Geometry: see drawing. Coordinates: mm, zero at the bounding-box minimum. Give positions to 0.01 mm unless a question says otherwise; leave off trailing zeros. Write each loop counter-clockwise with the first axis right and the second up, starting at its lowest first coordinate (ties: lowest second). Pieces come first, ordered by that corner, then holes. Notation, with made-up numbers: M -16,80 L 14,80 A18 cw 14,107 Z; hole C 78.25,-2.75 d2. An arc over 180 degrees is marked long. Use a Markdown table: item, result. Add a question column.
1) Section B-B on z = 1.8. Return the cut outline in (x, y) (1 decimal).
2) Pin query (flat end, axial travel): pin 1 (1 mm diameter, centred on x = 4.5, z = 0.5, fed in from +Y) (1 decimal); pin 2 (3.5 mm diameter, centred on x = 3, y = 3, fed in from +Z); pin 3 (2.5 mm diameter, centred on x = 8, y = 11, fed in from +Z). Return the tip coordinate at first contact, or that it passes through.
3) Section A-A on y = 3. Return the cut outline in (x, z), then the cut area to 3 significant figures.
4) Section C-C on x = 7.25. Return the cut outline in (y, z), then the cut area to 3 significant figures.
5) Draft query along Y for the marked faces 1, 2 and 3. Return one class per face: +Y half, -Y half, draft (parallel to the pull), parting line (faces both ways), or undercut.
6) Section D-D on y = 11. Return the cut outline in (x, z).
7) Line query: line 1 (X direction, y = 4, z = 0.85); line 2 (X direction, y = 10.75, z = 1.65); line 3 (X direction, y = 12.25, z = 1.5) (1 decimal). Output: solid intervals per line, ascending.
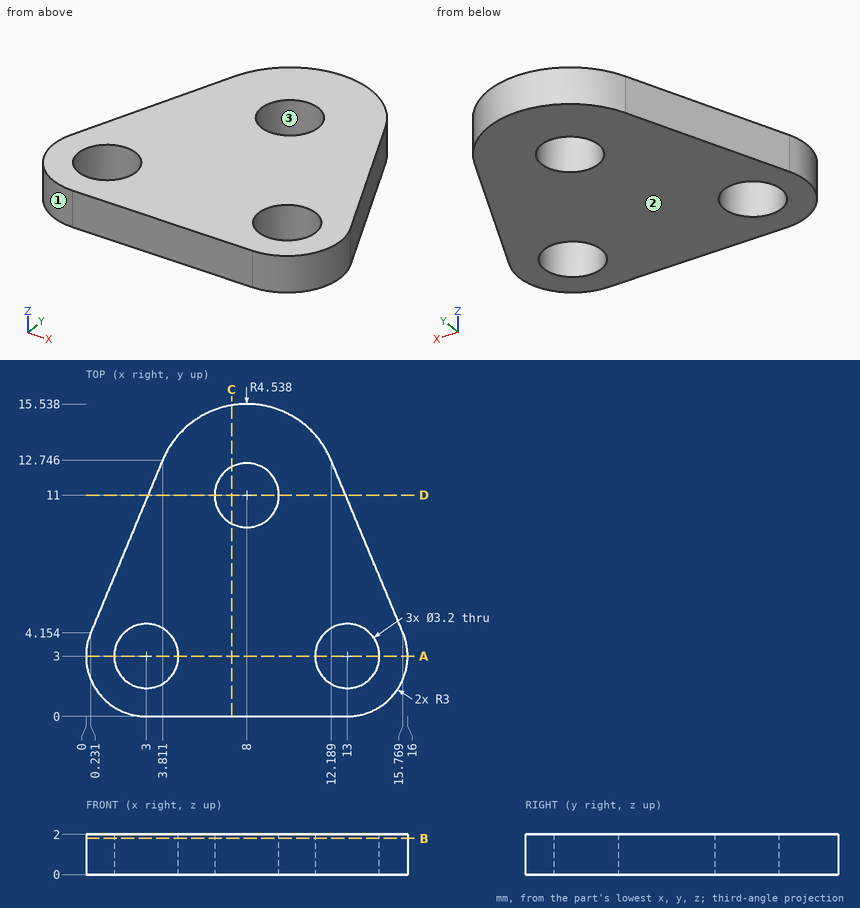
Found:
| question | item | result |
|---|---|---|
| 1 | outline | M 0.2,4.2 A3 ccw 3,0 L 13,0 A3 ccw 15.8,4.2 L 12.2,12.7 A4.5 ccw 3.8,12.7 Z; hole C 3,3 d3.2; hole C 8,11 d3.2; hole C 13,3 d3.2 |
| 2 | pin 1 | y = 14.4 |
| 2 | pin 2 | z = 2 |
| 2 | pin 3 | through |
| 3 | outline | M 0,0 L 1.4,0 L 1.4,2 L 0,2 Z; M 4.6,0 L 11.4,0 L 11.4,2 L 4.6,2 Z; M 14.6,0 L 16,0 L 16,2 L 14.6,2 Z |
| 3 | area | 19.2 mm² |
| 4 | outline | M 0,0 L 9.59,0 L 9.59,2 L 0,2 Z; M 12.41,0 L 15.48,0 L 15.48,2 L 12.41,2 Z |
| 4 | area | 25.3 mm² |
| 5 | face 1 | parting line |
| 5 | face 2 | draft |
| 5 | face 3 | undercut |
| 6 | outline | M 3.08,0 L 6.4,0 L 6.4,2 L 3.08,2 Z; M 9.6,0 L 12.92,0 L 12.92,2 L 9.6,2 Z |
| 7 | line 1 | 0.17 to 1.75, 4.25 to 11.75, 14.25 to 15.83 |
| 7 | line 2 | 2.98 to 6.42, 9.58 to 13.02 |
| 7 | line 3 | 3.6 to 7, 9 to 12.4 |
